from build123d import *

# Parameters (mm, degrees)
SKETCH1_W           = 6.35
SKETCH1_H           = 3.175
SKETCH1_W_2         = 3.175
SKETCH1_H_2         = 6.35
BOSS_EXTRUDE1_DEPTH = 3.175


with BuildPart() as part:
    # Sketch1 → Boss-Extrude1 (new body)
    with BuildSketch(Plane.XY):
        Polygon((0, 268.0208), (81, 268.0208), (81, 257.175), (84.175, 257.175), (84.175, 231.775), (81, 231.775), (81, 206.375), (84.175, 206.375), (84.175, 180.975), (81, 180.975), (81, 155.575), (84.175, 155.575), (84.175, 130.175), (81, 130.175), (81, 104.775), (84.175, 104.775), (84.175, 79.375), (81, 79.375), (81, 53.975), (84.175, 53.975), (84.175, 42.175), (-3.175, 42.175), (-3.175, 53.975), (0, 53.975), (0, 79.375), (-3.175, 79.375), (-3.175, 104.775), (0, 104.775), (0, 130.175), (-3.175, 130.175), (-3.175, 155.575), (0, 155.575), (0, 180.975), (-3.175, 180.975), (-3.175, 206.375), (0, 206.375), (0, 231.775), (-3.175, 231.775), (-3.175, 257.175), (0, 257.175), align=None)
        with Locations((53.2, 91.7575)):
            Rectangle(SKETCH1_W, SKETCH1_H, mode=Mode.SUBTRACT)
        with Locations((40.5, 91.7575)):
            Rectangle(SKETCH1_W, SKETCH1_H, mode=Mode.SUBTRACT)
        with Locations((65.9, 91.7575)):
            Rectangle(SKETCH1_W, SKETCH1_H, mode=Mode.SUBTRACT)
        with Locations((27.8, 91.7575)):
            Rectangle(SKETCH1_W, SKETCH1_H, mode=Mode.SUBTRACT)
        with Locations((15.1, 91.7575)):
            Rectangle(SKETCH1_W, SKETCH1_H, mode=Mode.SUBTRACT)
        with Locations((40.5, 160.02)):
            Rectangle(SKETCH1_W_2, SKETCH1_H_2, mode=Mode.SUBTRACT)
        with Locations((40.5, 172.72)):
            Rectangle(SKETCH1_W_2, SKETCH1_H_2, mode=Mode.SUBTRACT)
    extrude(amount=BOSS_EXTRUDE1_DEPTH)


solid = part.part
Verification items for the finished model (mm, model axes). Give positions to 0.01 mm unless a question says otherwise; leave off trailing zeros. Loops run counter-clockwise (first coordinate to the right, second up) from the corner with the lowest first, then second, coordinate; pieces in that order, holes last.
1. Go/stop test with a flat-tipped pin: P1, Ø1.5, axis at y = 159, z = 1, coming from the +X side. Record where the tip stops, or that it passes through.
Derived:
P1: stops at x = 81
2. Material ranges on probe 1 along Y at (x, z) = (41.5, 3.05) (3 decimals); probe 2 along Y at (x, z) = (12, 1.55) (3 decimals); probe 3 along X at (y, z) = (110, 2.4), recorded low to high.
Derived:
probe 1: y = 42.175 to 90.17, 93.345 to 156.845, 163.195 to 169.545, 175.895 to 268.021
probe 2: y = 42.175 to 90.17, 93.345 to 268.021
probe 3: x = 0 to 81
3. Cross-section at B-B on z = 0.5. Count the separate pieces of the cut face and the enclosed holes in it, and give its area (3 significant figures).
Derived:
separate pieces: 1
enclosed holes: 7
area: 18,900 mm2
4. Cross-section at A-A on y = 226. Record the cut outline in (x, z) (3 decimals), and give its area (3 significant figures).
Derived:
outline: (0, 0) - (81, 0) - (81, 3.175) - (0, 3.175) - close
area: 257 mm2
